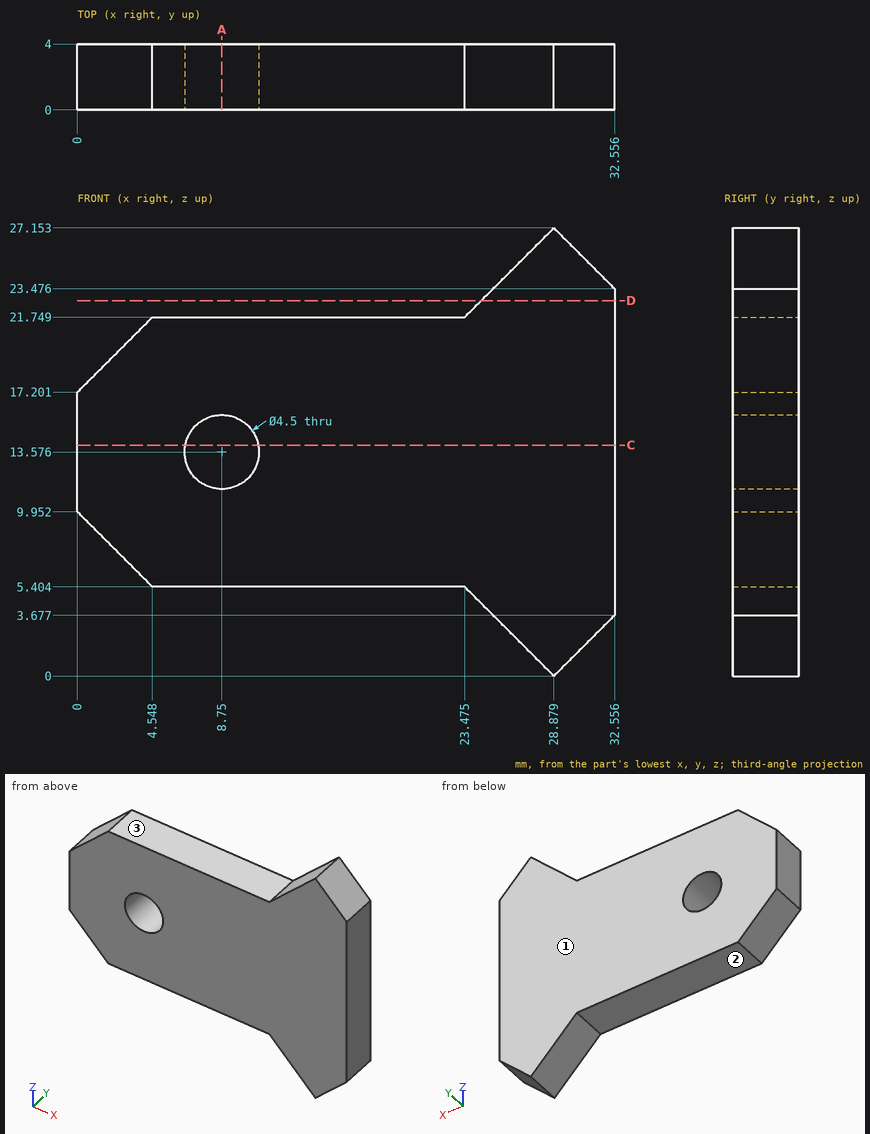
Drawing for the job (mm, zero at the part's lowest x, y, z). A direction names the side the tool comes from. Give positions to 0.01 mm unless a question says otherwise; leave off trailing zeros. Order: outer loops, then holes, each group sorted by start corner. A loop starts at its lowest first (then second) coordinate and runs counter-clockwise, first axis right, second up. Notation, with made-up numbers: (34.25, 38) - (86.25, 38) arc R20 ccw to (86.25, 52) - close; hole circle Ø4 at (20, 27). An arc over 180 degrees is marked (long way). Use one line per item in the form item = value.
Item 1: Pin check, flat tips, straight feed: pin 1 Ø5 at (x, z) = (6, 13) entering from -Y; pin 2 Ø1 at (y, z) = (0.5, 18.5) entering from -X; pin 3 Ø3.5 at (x, z) = (8.75, 13.58) entering from -Y; pin 4 Ø2 at (x, y) = (16.5, 3) entering from -Z. Stop position of each tip, or through.
Solution:
pin_1 = 0
pin_2 = 0.8
pin_3 = through
pin_4 = 5.4
Item 2: Slice it at C-C on z = 14. Give the cut face in (x, y).
Solution:
outline = (0, 0) - (6.54, 0) - (6.54, 4) - (0, 4) - close; (10.96, 0) - (32.56, 0) - (32.56, 4) - (10.96, 4) - close
Item 3: Slice it at D-D on z = 22.75. Give the cut face in (x, y), and give its area (3 significant figures).
Solution:
outline = (24.48, 0) - (32.56, 0) - (32.56, 4) - (24.48, 4) - close
area = 32.3 mm2
Item 4: Slice it at A-A on x = 8.75. Give the cut face in (y, z) (1 decimal).
Solution:
outline = (0, 5.4) - (4, 5.4) - (4, 11.3) - (0, 11.3) - close; (0, 15.8) - (4, 15.8) - (4, 21.7) - (0, 21.7) - close
Item 5: Probe probe 1 along Z at (x, y) = (11.5, 2.35) (1 decimal); probe 2 along X at (y, z) = (1.6, 14.5) (1 decimal); probe 3 along X at (y, z) = (1.9, 14.75) (1 decimal). List the from-to ranges inside material, lowest first. Write a range as from..to.
Solution:
probe_1 = 5.4..21.7
probe_2 = 0..6.7, 10.8..32.6
probe_3 = 0..6.8, 10.7..32.6
Item 6: Which spindle directions (+Z, -Z, +X, -X, +Y, -Y) get a long thin tool onto all of the face, cutting with end or side? Do the marked faces 1, 2 and 3. Say none if no direction does.
Solution:
face_1 = +Z, -Z, +X, -X, +Y
face_2 = -Z, -X, +Y, -Y
face_3 = +Z, -X, +Y, -Y
